from build123d import *

# Parameters (mm, degrees)
SKETCH1_W           = 3
SKETCH1_H           = 2.75
SKETCH2_R           = 1.5
BOSS_EXTRUDE1_DEPTH = 45
CUT_EXTRUDE1_DEPTH  = 1.5
CHAMFER1_SIZE       = 0.3


with BuildPart() as part:
    # Sketch1 → Revolve1 (revolve)
    with BuildSketch(Plane.XY, mode=Mode.PRIVATE) as revolve1_sk:
        with Locations((-1.5, 1.375)):
            Rectangle(SKETCH1_W, SKETCH1_H)
    revolve(revolve1_sk.sketch.rotate(Axis((-3, 0, 0), (1, 0, 0)), 270), axis=Axis((-3, 0, 0), (1, 0, 0)))

    # Sketch2 → Boss-Extrude1 (add)
    with BuildSketch(Plane(origin=(0, 0, 0), x_dir=(0, 0, -1), z_dir=(1, 0, 0))):
        with Locations(Location((0, 0, 0), (0, 0, 180))):
            Circle(SKETCH2_R)
    extrude(amount=BOSS_EXTRUDE1_DEPTH)

    # Sketch3 → Cut-Extrude1 (cut)
    with BuildSketch(Plane.ZY.offset(3)):
        Polygon((1.25, -0.721687836), (1.25, 0.721687836), (0, 1.443375673), (-1.25, 0.721687836), (-1.25, -0.721687836), (0, -1.443375673), align=None)
    extrude(amount=-CUT_EXTRUDE1_DEPTH, mode=Mode.SUBTRACT)

    # Sketch4 → Cut-Revolve1 (revolve, cut)
    with BuildSketch(Plane.XY, mode=Mode.PRIVATE) as cut_revolve1_sk:
        Polygon((-1.5, 1.25), (-1.5, 0), (-1.165063509, 0), align=None)
    revolve(cut_revolve1_sk.sketch.rotate(Axis((-1.500025, 0, 0), (1, 0, 0)), 90), axis=Axis((-1.500025, 0, 0), (1, 0, 0)), mode=Mode.SUBTRACT)

    # Chamfer1
    chamfer1_edges = [part.edges().sort_by_distance(p)[0] for p in [
        (-3, 0, 2.75),
        (45, 0, -1.5),
    ]]
    chamfer(chamfer1_edges, length=CHAMFER1_SIZE)


solid = part.part
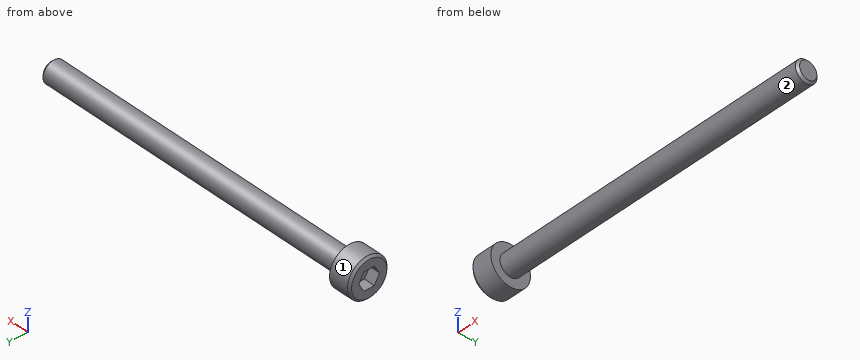
Check sheet for the modelled part. Datum: model origin and axes. Units: mm. Face numbers are marked on the shaded views. A direction names the side the tool comes from. Give positions to 0.01 mm unless a question says otherwise; leave off trailing zeros. Order: outer loops, then holes, each group sorted by start corner. A loop starts at its lowest first (then second) coordinate and runs counter-clockwise, first axis right, second up. Notation, with made-up numbers: M -29,-21 L 11,-21 A26 ccw 11,15 Z; hole C 8,81.25 d1. An arc over 180 degrees is marked long. Answer as CSV lines item,"result". Start each with the question number.
Item 1: Thickness scan on line 1 (X direction, y = 1.6, z = -1.8); line 2 (Z direction, x = 43.5, y = -0.4); line 3 (Y direction, x = 19, z = 0). Record the ranges inside material, lowest first. Write a range as [from, to].
Item 2: Cross-section at A-A on x = 23. Enter the section's corners in (y, z).
Item 3: Tool access check on the marked faces 1 and 2. Record the directions out of +Z, -Z, +X, -X, +Y, -Y that give a thin tool (end or side, any length) a straight path to the whole face; none if there is none.
Item 4: Gauge pin test, flat ends, axial feed: P1, Ø1, axis at x = 30.5, y = -0.5, coming from the +Z side; P2, Ø1.5, axis at x = 30, y = -1.5, coming from the -Z side; P3, Ø1, axis at x = 37.5, z = -0.5, coming from the -Y side. Record the tip position at first contact, or that the pin passes through.
Established:
1,line 1,"x = [-3, 0]"
1,line 2,"z = [-1.45, 1.45]"
1,line 3,"y = [-1.5, 1.5]"
2,outline,"C 0,0 d3"
3,face 1,"+X, -X"
3,face 2,"+X"
4,P1,"stops at z = 1.5"
4,P2,"stops at z = -1.3"
4,P3,"stops at y = -1.5"
